Part model, mm, in its own coordinate system. A direction names the side the tool comes from. Round coordinates to 2 decimals unless told otherwise and drop trailing zeros. Write each loop counter-clockwise with the first axis right and the second up, starting at its lowest first coordinate (ties: lowest second). Pieces come first, ordered by that corner, then holes. Notation, with made-up numbers: (51, 50) -> (64, 50) arc R9 ccw to (64, 60) -> close; hole circle Ø7 at (-6, 86.5). An arc over 180 degrees is marked (long way). Use CSV: the item, a comma, the result in double quotes. Start each with the question number.
(1) Which spindle directions (+Z, -Z, +X, -X, +Y, -Y) get a long thin tool onto all of the face, cutting with end or side? Do faces 4 (the cylindrical face through (0.805, 14.246, 10.684)), 5 (the flat face through (13, 1.587, 116)), 6 (the cylindrical face through (12.812, 24.617, 218.125)). Say none if no direction does.
(2) Saw through at A-A (y = 18.5). Give the cut face in (x, z).
(3) Saw through at C-C (z = 216). Give the cut face in (x, y).
(4) Probe line 1 (Y direction, x = 11.5, z = 114.5); line 2 (Y direction, x = 0.6, z = 12.7). List the from-to ranges inside material, lowest first. Write a range as [from, to].
(5) Two-plate mould, pull along Y, no slides. Class faces 1 (the flat face through (13, 0, 116)), 2 (the cylindrical face through (0.805, 13.463, 219.827)), 3 (the cylindrical face through (15.22, 24.62, 13.96)): released by +Y, released by -Y, zero draft, split by the parting line, or undercut.
```python
from build123d import *

# Parameters (mm, degrees)
SKETCH1_W           = 25.4
SKETCH1_H           = 25.4
SKETCH1_W_2         = 22.225
SKETCH1_H_2         = 22.225
BOSS_EXTRUDE1_DEPTH = 234.95
SKETCH4_R           = 2.54
CUT_EXTRUDE3_DEPTH  = 238.680084357
CUT_EXTRUDE4_REACH  = 239.68
SKETCH5_R           = 2.54


with BuildPart() as part:
    # Sketch1 → Boss-Extrude1 (new body)
    with BuildSketch(Plane.XY):
        with Locations((12.7, 12.7)):
            Rectangle(SKETCH1_W, SKETCH1_H)
        with Locations((12.7, 12.7)):
            Rectangle(SKETCH1_W_2, SKETCH1_H_2, mode=Mode.SUBTRACT)
    extrude(amount=BOSS_EXTRUDE1_DEPTH)

    # Sketch4 → Cut-Extrude3 (cut, through all)
    with BuildSketch(Plane(origin=(25.4, 0, 0), x_dir=(0, 0, -1), z_dir=(1, 0, 0))):
        with Locations((-222.25, 12.7)):
            Circle(SKETCH4_R)
        with Locations((-196.85, 12.7)):
            Circle(SKETCH4_R)
        with Locations(Location((-38.1, 12.7, 0), (0, 0, 180))):
            Circle(SKETCH4_R)
        with Locations(Location((-12.7, 12.7, 0), (0, 0, 180))):
            Circle(SKETCH4_R)
        with Locations((-104.775, 12.7)):
            Circle(SKETCH4_R)
        with Locations(Location((-130.175, 12.7, 0), (0, 0, 180))):
            Circle(SKETCH4_R)
    extrude(amount=-CUT_EXTRUDE3_DEPTH, mode=Mode.SUBTRACT)

    # Sketch5 → Cut-Extrude4 (cut, up to next)
    with BuildSketch(Plane(origin=(0, 25.4, 0), x_dir=(1, 0, 0), z_dir=(0, 1, 0)), mode=Mode.PRIVATE) as cut_extrude4_sk1:
        with Locations(Location((12.7, -220.6625, 0), (0, 0, 270))):
            Circle(SKETCH5_R)
    cut_extrude4_tool1 = extrude(cut_extrude4_sk1.sketch, amount=-CUT_EXTRUDE4_REACH, mode=Mode.PRIVATE) & part.part
    # Sketch5 → Cut-Extrude4 (cut, up to next)
    with BuildSketch(Plane(origin=(0, 25.4, 0), x_dir=(1, 0, 0), z_dir=(0, 1, 0)), mode=Mode.PRIVATE) as cut_extrude4_sk2:
        with Locations(Location((12.7, -14.2875, 0), (0, 0, 270))):
            Circle(SKETCH5_R)
    cut_extrude4_tool2 = extrude(cut_extrude4_sk2.sketch, amount=-CUT_EXTRUDE4_REACH, mode=Mode.PRIVATE) & part.part
    add(cut_extrude4_tool1.solids().sort_by_distance((12.7, 25.4, 220.6625))[0], mode=Mode.SUBTRACT)
    add(cut_extrude4_tool2.solids().sort_by_distance((12.7, 25.4, 14.2875))[0], mode=Mode.SUBTRACT)


solid = part.part
```
Answers:
1,face 4,"+X, -X"
1,face 5,"+Z, -Z"
1,face 6,"+Y"
2,outline,"(0, 0) -> (1.59, 0) -> (1.59, 234.95) -> (0, 234.95) -> close; (23.81, 0) -> (25.4, 0) -> (25.4, 234.95) -> (23.81, 234.95) -> close"
3,outline,"(0, 0) -> (25.4, 0) -> (25.4, 25.4) -> (0, 25.4) -> close; hole (1.59, 1.59) -> (23.81, 1.59) -> (23.81, 23.81) -> (1.59, 23.81) -> close"
4,line 1,"y = [0, 1.59], [23.81, 25.4]"
4,line 2,"y = [0, 10.16], [15.24, 25.4]"
5,face 1,"released by -Y"
5,face 2,"undercut"
5,face 3,"zero draft"
